Geometry check sheet. Reference: drawing and pictorial views, mm from the part's lowest x, y, z. Give positions to 0.01 mm unless a question says otherwise; leave off trailing zeros. Order: outer loops, then holes, each group sorted by start corner. A loop starts at its lowest first (then second) coordinate and runs counter-clockwise, first axis right, second up.
Item 1: Sectioned sample at D-D on x = 10. Record the boundary of the cut face in (y, z).
Item 2: Sectioned sample at A-A on x = 110. Record the boundary of the cut face in (y, z).
Item 3: Sectioned sample at B-B on y = 11. Record the boundary of the cut face in (x, z), and give its area (3 significant figures).
Item 4: Material ranges on line 1 along Y through (x, z) = (23.5, 5.75); line 2 along Y through (x, z) = (110, 7.5); line 3 along X through (y, z) = (10.5, 3.25) (1 decimal), recorded low to high.
Item 5: Gauge pin test, flat ends, axial feed: P1, Ø5.5, axis at x = 22.5, y = 12, coming from the +Z side; P2, Ø3.5, axis at x = 23.5, y = 11, coming from the +Z side. Record the tip position at first contact, or that the pin passes through.
Item 6: Sectioned sample at C-C on z = 1.75. Record the boundary of the cut face in (x, y) (1 decimal).
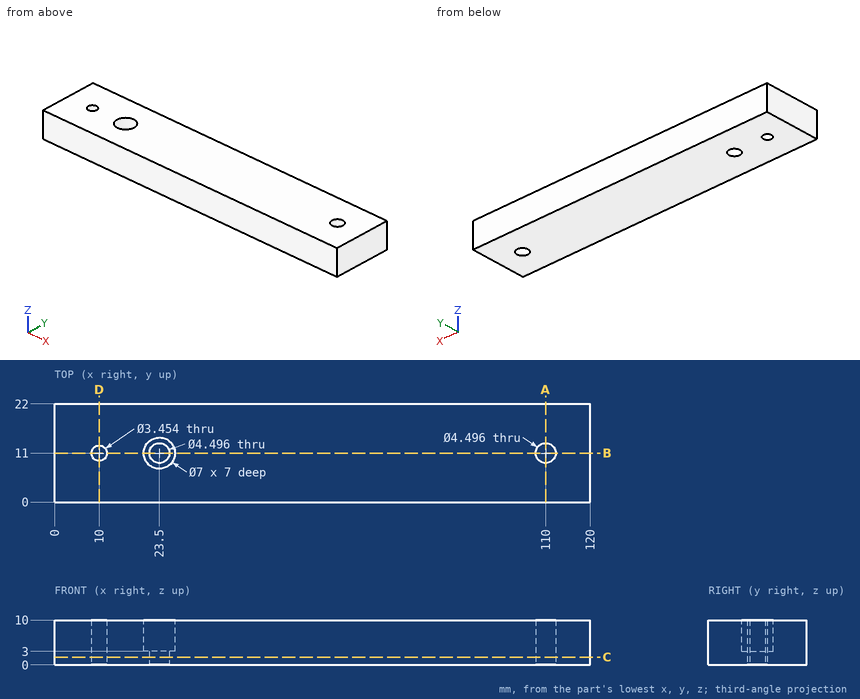
Report:
1. outline: (0, 0) - (9.27, 0) - (9.27, 10) - (0, 10) - close; (12.73, 0) - (22, 0) - (22, 10) - (12.73, 10) - close
2. outline: (0, 0) - (8.75, 0) - (8.75, 10) - (0, 10) - close; (13.25, 0) - (22, 0) - (22, 10) - (13.25, 10) - close
3. outline: (0, 0) - (8.27, 0) - (8.27, 10) - (0, 10) - close; (11.73, 0) - (21.25, 0) - (21.25, 3) - (20, 3) - (20, 10) - (11.73, 10) - close; (25.75, 0) - (107.75, 0) - (107.75, 10) - (27, 10) - (27, 3) - (25.75, 3) - close; (112.25, 0) - (120, 0) - (120, 10) - (112.25, 10) - close
3. area: 1,060 mm2
4. line 1: y = 0 to 7.5, 14.5 to 22
4. line 2: y = 0 to 8.75, 13.25 to 22
4. line 3: x = 0 to 8.3, 11.7 to 20, 27 to 107.8, 112.2 to 120
5. P1: stops at z = 10
5. P2: passes through
6. outline: (0, 0) - (120, 0) - (120, 22) - (0, 22) - close; hole circle Ø3.5 at (10, 11); hole circle Ø4.5 at (23.5, 11); hole circle Ø4.5 at (110, 11)
